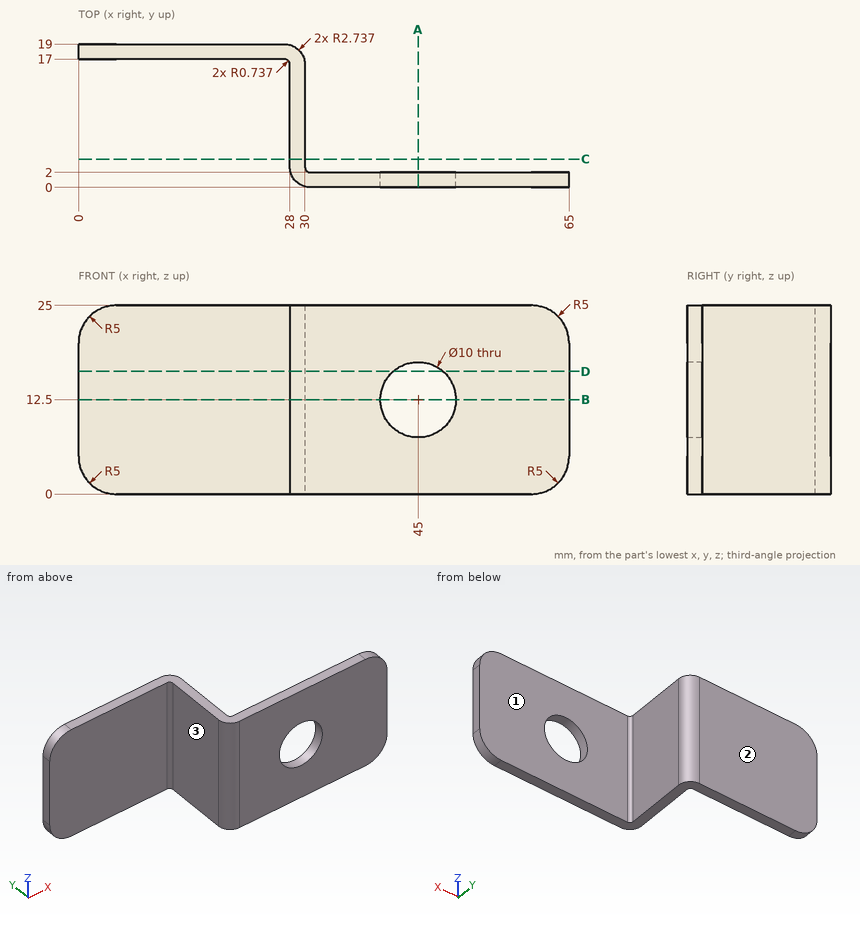
Part print with two shaded views. Sizes in mm from the minimum x, y, z corner. A direction names the side the tool comes from. Round coordinates to 2 decimals unless told otherwise and drop trailing zeros. Order: outer loops, then holes, each group sorted by start corner. A loop starts at its lowest first (then second) coordinate and runs counter-clockwise, first axis right, second up.
(1) Drill centre lines: line 1 (Y direction, x = 53.5, z = 4.5); line 2 (Y direction, x = 11, z = 14.75); line 3 (X direction, y = 0.65, z = 12.5) (1 decimal). Where is each one in solid material? Low to high.
(2) Band-saw the part on D-D (z = 16.25). List the corners of the cut face in (x, y).
(3) Band-saw the part on C-C (y = 3.75). List the corners of the cut face in (x, z).
(4) Pin check, flat tips, straight feed: pin 1 (1.5 mm diameter, centred on y = 13.5, z = 11, fed in from -X); pin 2 (5 mm diameter, centred on x = 49.5, z = 5, fed in from +Y); pin 3 (8 mm diameter, centred on y = 7.5, z = 6.5, fed in from +X). Stop position of each tip, or through.
(5) Band-saw the part on A-A (x = 45). List the corners of the cut face in (y, z), then the cut area to 3 significant figures.
(6) Band-saw the part on B-B (z = 12.5). List the corners of the cut face in (x, y).
(7) 3-axis set-ups, long thin cutter, end or side, ignore diameter. For the marked faces 1, 2 and 3: which of +Z, -Z, +X, -X, +Y, -Y reach the whole face in a straight line?
Verdict:
1. line 1: y = 0 to 2
1. line 2: y = 17 to 19
1. line 3: x = 29 to 40, 50 to 65
2. outline: (0, 17) - (27.26, 17) arc R0.74 cw to (28, 16.26) - (28, 2.74) arc R2.74 ccw to (30.74, 0) - (41.69, 0) - (41.69, 2) - (30.74, 2) arc R0.74 cw to (30, 2.74) - (30, 16.26) arc R2.74 ccw to (27.26, 19) - (0, 19) - close; (48.31, 0) - (65, 0) - (65, 2) - (48.31, 2) - close
3. outline: (28, 0) - (30, 0) - (30, 25) - (28, 25) - close
4. pin 1: stops at x = 28
4. pin 2: stops at y = 2
4. pin 3: stops at x = 30
5. outline: (0, 0) - (2, 0) - (2, 7.5) - (0, 7.5) - close; (0, 17.5) - (2, 17.5) - (2, 25) - (0, 25) - close
5. area: 30.0 mm2
6. outline: (0, 17) - (27.26, 17) arc R0.74 cw to (28, 16.26) - (28, 2.74) arc R2.74 ccw to (30.74, 0) - (40, 0) - (40, 2) - (30.74, 2) arc R0.74 cw to (30, 2.74) - (30, 16.26) arc R2.74 ccw to (27.26, 19) - (0, 19) - close; (50, 0) - (65, 0) - (65, 2) - (50, 2) - close
7. face 1: +Z, -Z, +X, +Y
7. face 2: +Z, -Z, +X, -X, +Y
7. face 3: +Z, -Z, -X, -Y
